```python
from build123d import *

# Parameters (mm, degrees)
EXTRUDE1_DEPTH     = 25.4
SKETCH11_R         = 11.1125
CUT_EXTRUDE4_DEPTH = 133.202058985
SKETCH12_R         = 4.953
CUT_EXTRUDE5_DEPTH = 133.202058985
SKETCH13_R         = 3.2639
CUT_EXTRUDE6_DEPTH = 137.930502446


with BuildPart() as part:
    # Sketch1 → Extrude1 (new, symmetric)
    with BuildSketch(Plane.XY):
        with BuildLine():
            Line((0, 127), (0, 0))
            Line((0, 0), (-50.8, 0))
            Line((-50.8, 0), (-50.8, 0.254))
            ThreePointArc((-50.8, 0.254), (-49.425137622, 4.11043301), (-45.920710119, 6.227343493))
            Line((-45.920710119, 6.227343493), (-12.703242032, 12.993408361))
            ThreePointArc((-12.703242032, 12.993408361), (-8.140185388, 15.74980222), (-6.35, 20.771199368))
            Line((-6.35, 20.771199368), (-6.35, 120.904))
            ThreePointArc((-6.35, 120.904), (-4.564522938, 125.214522938), (-0.254, 127))
            Line((-0.254, 127), (0, 127))
        make_face()
    extrude(amount=EXTRUDE1_DEPTH, both=True)

    # Sketch11 → Cut-Extrude4 (cut, through all)
    with BuildSketch(Plane(origin=(0, 7.62, 0), x_dir=(-1, 0, 0), z_dir=(0, 1, 0))):
        with Locations((33.3248, -12.7)):
            Circle(SKETCH11_R)
        with Locations((33.3248, 12.7)):
            Circle(SKETCH11_R)
    extrude(amount=CUT_EXTRUDE4_DEPTH, mode=Mode.SUBTRACT)

    # Sketch12 → Cut-Extrude5 (cut, through all)
    with BuildSketch(Plane(origin=(0, 7.62, 0), x_dir=(-1, 0, 0), z_dir=(0, 1, 0))):
        with Locations(Location((33.3248, 12.7, 0), (0, 0, 90))):
            Circle(SKETCH12_R)
        with Locations(Location((33.3248, -12.7, 0), (0, 0, 90))):
            Circle(SKETCH12_R)
    extrude(amount=-CUT_EXTRUDE5_DEPTH, mode=Mode.SUBTRACT)

    # Sketch13 → Cut-Extrude6 (cut, through all)
    with BuildSketch(Plane.ZY.offset(6.35)):
        with Locations(Location((-12.7, 69.85, 0), (0, 0, 270))):
            Circle(SKETCH13_R)
        with Locations(Location((-12.7, 107.95, 0), (0, 0, 270))):
            Circle(SKETCH13_R)
        with Locations(Location((12.7, 107.95, 0), (0, 0, 270))):
            Circle(SKETCH13_R)
        with Locations(Location((12.7, 69.85, 0), (0, 0, 270))):
            Circle(SKETCH13_R)
    extrude(amount=-CUT_EXTRUDE6_DEPTH, mode=Mode.SUBTRACT)


solid = part.part
```
Could you check a few things on this model? Use its own coordinates, in mm. A direction names the side the tool comes from. Coordinates: 2 decimals unless noted, no trailing zeros. Order: outer loops, then holes, each group sorted by start corner. A loop starts at its lowest first (then second) coordinate and runs counter-clockwise, first axis right, second up. Notation, with made-up numbers: M -21,58.5 L 1,58.5 A17 cw 1,86.5 Z; hole C 45,27.5 d2. An arc over 180 degrees is marked long. Use a Markdown table: item, result. Add a question column.
Q1. I want a section at B-B on y = 69.85. List the corners of the cut face in (x, z) for me, then the cut area to 3 significant figures.
Q2. We'd pull the mould along Y, two halves only. Please class faces 4 (the flat face through (0, 64, 0)), 5 (the cylindrical face through (-3.22, 73.11, 12.84)), 6 (the cylindrical face through (-8.19, 15.69, 0.36)), 7 (the flat face through (-25, 0, 0)): pulls with the +Y half, pulls with the -Y half, needs draft (parallel to the pull), parting line crosses it, or undercut.
Q3. If I drill on L1, parallel to Y at x = -2, z = 12; L2, parallel to Y at x = -3, z = 12; L3, parallel to X at y = 96, z = -14, over which ranges is the centre line in solid material (lowest first)?
Q4. I want a section at A-A on z = 12.7. Give the number of separate pieces and of enclosed holes in the cut face, then the cut area to 3 significant figures.
Q5. Which directions (+Z, -Z, +X, -X, +Y, -Y) give clear straight access to the entire face, cutting with the end or side of a thin tool? Please do faces 1 (the cylindrical face through (-3.219, 104.837, 13.68)), 2 (the cylindrical face through (-22.217, 8.968, 13.029)), 3 (the flat face through (-6.35, 70, 0)).
Q6. I want a section at D-D on x = -25.5. List the corners of the cut face in (y, z) for me.
Q7. I'm going to push flat-ended pins straight in: pin 1 (18.5 mm diameter, centred on x = -28.5, z = 7.5, fed in from +Y); pin 2 (12 mm diameter, centred on x = -40.5, z = 4, fed in from +Y); pin 3 (13 mm diameter, centred on x = -33.32, z = -12.7, fed in from +Y). Where does each tip first touch, or does it pass through?
Checked values:
| question | item | result |
|---|---|---|
| 1 | outline | M -6.35,-25.4 L 0,-25.4 L 0,-15.96 L -6.35,-15.96 Z; M -6.35,-9.44 L 0,-9.44 L 0,9.44 L -6.35,9.44 Z; M -6.35,15.96 L 0,15.96 L 0,25.4 L -6.35,25.4 Z |
| 1 | area | 240 mm² |
| 2 | face 4 | needs draft |
| 2 | face 5 | undercut |
| 2 | face 6 | pulls with the +Y half |
| 2 | face 7 | pulls with the -Y half |
| 3 | L1 | 0 to 66.66, 73.04 to 104.76, 111.14 to 126.74 |
| 3 | L2 | 0 to 66.66, 73.04 to 104.76, 111.14 to 126.35 |
| 3 | L3 | -6.35 to 0 |
| 4 | separate pieces | 4 |
| 4 | enclosed holes | 0 |
| 4 | area | 1,050 mm² |
| 5 | face 1 | +X, -X |
| 5 | face 2 | +Y |
| 5 | face 3 | +Z, -Z, -X, +Y |
| 6 | outline | M 0,-25.4 L 10.39,-25.4 L 10.39,-20.59 L 7.62,-20.59 L 7.62,-4.81 L 10.39,-4.81 L 10.39,4.81 L 7.62,4.81 L 7.62,20.59 L 10.39,20.59 L 10.39,25.4 L 0,25.4 Z |
| 7 | pin 1 | y = 11.66 |
| 7 | pin 2 | y = 8.46 |
| 7 | pin 3 | y = 7.62 |
